```python
from build123d import *

# Parameters (mm, degrees)
SKETCH2_R                 = 2.5
BOSS_EXTRUDE1_DEPTH       = 3.1
CUT_EXTRUDE1_DEPTH        = 14.7
CUT_EXTRUDE1_TAPER        = 2
SKETCH4_W                 = 2
SKETCH4_H                 = 12.7
F_2_CLEARANCE_HOLE1_D     = 2.360316922
F_2_CLEARANCE_HOLE1_DEPTH = 18.7
CHAMFER1_SIZE             = 0.25
FILLET1_R                 = 0.5


with BuildPart() as part:
    # Sketch1 → Revolve1 (revolve)
    with BuildSketch(Plane.XY):
        Polygon((3.95, 0), (0, 0), (0, -15.6), (3.6, -15.6), (3.6, -11.2), (4, -11.054411906), (4, -2.1), (2.2, -2.1), (2.2, -1.5), (3.95, -1.5), align=None)
    revolve(axis=Axis((0, 0, 0), (0, -1, 0)))

    # Sketch2 → Boss-Extrude1 (add)
    with BuildSketch(Plane.XZ.offset(15.6)):
        Circle(SKETCH2_R)
    extrude(amount=BOSS_EXTRUDE1_DEPTH)

    # Sketch3 → Cut-Extrude1 (cut)
    with BuildSketch(Plane(origin=(0, 0, 0), x_dir=(-1, 0, 0), z_dir=(0, 1, 0))):
        Polygon((0.977739085, -1.693493773), (1.955478171, 0), (0.977739085, 1.693493773), (-0.977739085, 1.693493773), (-1.955478171, 0), (-0.977739085, -1.693493773), align=None)
    extrude(amount=-CUT_EXTRUDE1_DEPTH, taper=CUT_EXTRUDE1_TAPER, mode=Mode.SUBTRACT)

    # Sketch4 → Cut-Revolve1 (revolve, cut)
    with BuildSketch(Plane(origin=(0, 0, 0), x_dir=(0, 0, -1), z_dir=(1, 0, 0))):
        with Locations((-1, -6.35)):
            Rectangle(SKETCH4_W, SKETCH4_H)
    revolve(axis=Axis((0, -12.7, 0), (0, 1, 0)), mode=Mode.SUBTRACT)

    # #2 Clearance Hole1
    with Locations(Plane(origin=(0, -18.7, 0), x_dir=(-1, 0, 0), z_dir=(0, -1, 0))):
        with Locations((0, 0)):
            Hole(F_2_CLEARANCE_HOLE1_D / 2, depth=F_2_CLEARANCE_HOLE1_DEPTH)

    # Chamfer1
    chamfer1_edges = [part.edges().sort_by_distance(p)[0] for p in [
        (-2.5, -18.7, 0),
    ]]
    chamfer(chamfer1_edges, length=CHAMFER1_SIZE)

    # Fillet1
    fillet1_edges = [part.edges().sort_by_distance(p)[0] for p in [
        (-3.95, 0, 0),
        (0, 0, -2),
    ]]
    fillet(fillet1_edges, radius=FILLET1_R)


solid = part.part
```
Work out the finished part from the listing and answer in its coordinate system (mm). A direction names the side the tool comes from. Give positions to 0.01 mm unless a question says otherwise; leave off trailing zeros. Order: outer loops, then holes, each group sorted by start corner. A loop starts at its lowest first (then second) coordinate and runs counter-clockwise, first axis right, second up. Notation, with made-up numbers: (43.25, 18.5) - (99.25, 18.5) arc R8 ccw to (99.25, 33.5) - close; hole circle Ø4 at (8, -29). An arc over 180 degrees is marked (long way). One line per item, written item: value. Start each with the question number.
1. Consider line 1 (Z direction, x = 0, y = -15.55); line 2 (Z direction, x = 0, y = -17.25); line 3 (Y direction, x = -0.5, z = -3.25). Determine where each line is inside the solid, lowest interval first.
2. Which of the six approach directions +Z, -Z, +X, -X, +Y, -Y give full straight-line access (tool end or side, diameter ignored) to faces 4 (the face through (-0.54, -17.01, -2.44)), 5 (the face through (2.1, -1.8, 0.66)), 6 (the face through (-2, -7, 0))?
3. Section A-A, the plane y = -10.75 is taken. Write down the section's boundary in (x, z).
4. For a pull along Y with two mould halves and no side action, classify faces 1 (the face through (0.9, -15.6, 2.5)), 2 (the face through (3.434, -13.369, 1.081)), 3 (the face through (2, -2.1, -2)) as released by +Y, released by -Y, zero draft, split by the parting line, or undercut.
Filled sheet:
1. line 1: -3.6 to -1.18, 1.18 to 3.6
1. line 2: -2.5 to -1.18, 1.18 to 2.5
1. line 3: -15.6 to -2.1, -1.5 to 0
2. face 4: -Y
2. face 5: none
2. face 6: +Y
3. outline: circle Ø8 at (0, 0); hole circle Ø4 at (0, 0)
4. face 1: released by -Y
4. face 2: zero draft
4. face 3: undercut
